```python
from build123d import *

# Parameters (mm, degrees)
F1_R     = 5
F1_R_2   = 1.5
F2_DEPTH = 1
F3_R     = 0.2


with BuildPart() as f2:
    # F1 (on offset) → F2 (new body)
    with BuildSketch(Plane.XY):
        Circle(F1_R)
        Circle(F1_R_2, mode=Mode.SUBTRACT)
    extrude(amount=F2_DEPTH)

    # F3
    f3_edges = [f2.edges().sort_by_distance(p)[0] for p in [
        (-5, 0, 1),
        (-1.5, 0, 1),
        (-5, 0, 0),
        (-1.5, 0, 0),
    ]]
    fillet(f3_edges, radius=F3_R)


solid = f2.part
```
Here's how the part is built. I have some questions about the finished solid (model axes, mm). Give positions to 0.01 mm unless a question says otherwise; leave off trailing zeros. Write each loop counter-clockwise with the first axis right and the second up, starting at its lowest first coordinate (ties: lowest second). Pieces come first, ordered by that corner, then holes. Notation, with made-up numbers: M -1,-27.75 L 30,-27.75 A11 cw 30,-17.75 Z; hole C 86,16.5 d1. An arc over 180 degrees is marked long. Put each result on its own line as item: value. Start each with the question number.
Item 1: Thinking about a two-plate mould opening in Y: for faces 1 (the cylindrical face through (-1.08, -4.88, 0.5)), 2 (the flat face through (2, 0, 0)), 3 (the cylindrical face through (-1.5, 0.07, 0.5)), which applies, +Y half, -Y half, draft (parallel to the pull), parting line (faces both ways), or undercut?
Item 2: If we section it at A-A, the plane y = 0: Write out the boundary of the cut face in (x, z), then the cut area to 3 significant figures.
Item 3: I need wall thicknesses on L1, parallel to Y at x = 0, z = 0.6; L2, parallel to Y at x = -0.5, z = 0.75; L3, parallel to X at y = 0.25, z = 0.4. Which ranges of each line are inside material? Lowest first, please. Write a range as from..to.
Values:
1. face 1: parting line
1. face 2: draft
1. face 3: undercut
2. outline: M -5,0.2 A0.2 ccw -4.8,0 L -1.7,0 A0.2 ccw -1.5,0.2 L -1.5,0.8 A0.2 ccw -1.7,1 L -4.8,1 A0.2 ccw -5,0.8 Z; M 1.5,0.2 A0.2 ccw 1.7,0 L 4.8,0 A0.2 ccw 5,0.2 L 5,0.8 A0.2 ccw 4.8,1 L 1.7,1 A0.2 ccw 1.5,0.8 Z
2. area: 6.93 mm²
3. L1: -5..-1.5, 1.5..5
3. L2: -4.97..-1.41, 1.41..4.97
3. L3: -4.99..-1.48, 1.48..4.99
